Print and shaded views of the part. All mm, measured from the part's lowest x, y and z. Coordinates: 2 decimals unless noted, no trailing zeros. Order: outer loops, then holes, each group sorted by start corner. A loop starts at its lowest first (then second) coordinate and runs counter-clockwise, first axis right, second up. Notation, with made-up numbers: (0.5, 42.25) -> (26.5, 42.25) arc R27 cw to (26.5, 81.25) -> close; hole circle Ø4 at (-23.75, 34.25). An arc over 180 degrees is marked (long way). Return JSON: item names as keys, results as strings. Group by question number.
1) Cut at D-D (z = 4). Write the cut outline in (x, y).
2) Cut at C-C (y = 0.2). State how many separate pieces and enclosed holes the cut face has, and give its area (3 significant figures).
3) Probe line 1 (Z direction, x = 10.5, y = 0.65); line 2 (Z direction, x = 36, y = 0.9). List the from-to ranges inside material, lowest first.
4) Cut at A-A (z = 12.5). Write the cut outline in (x, y).
5) Cut at B-B (x = 6). Write the cut outline in (y, z).
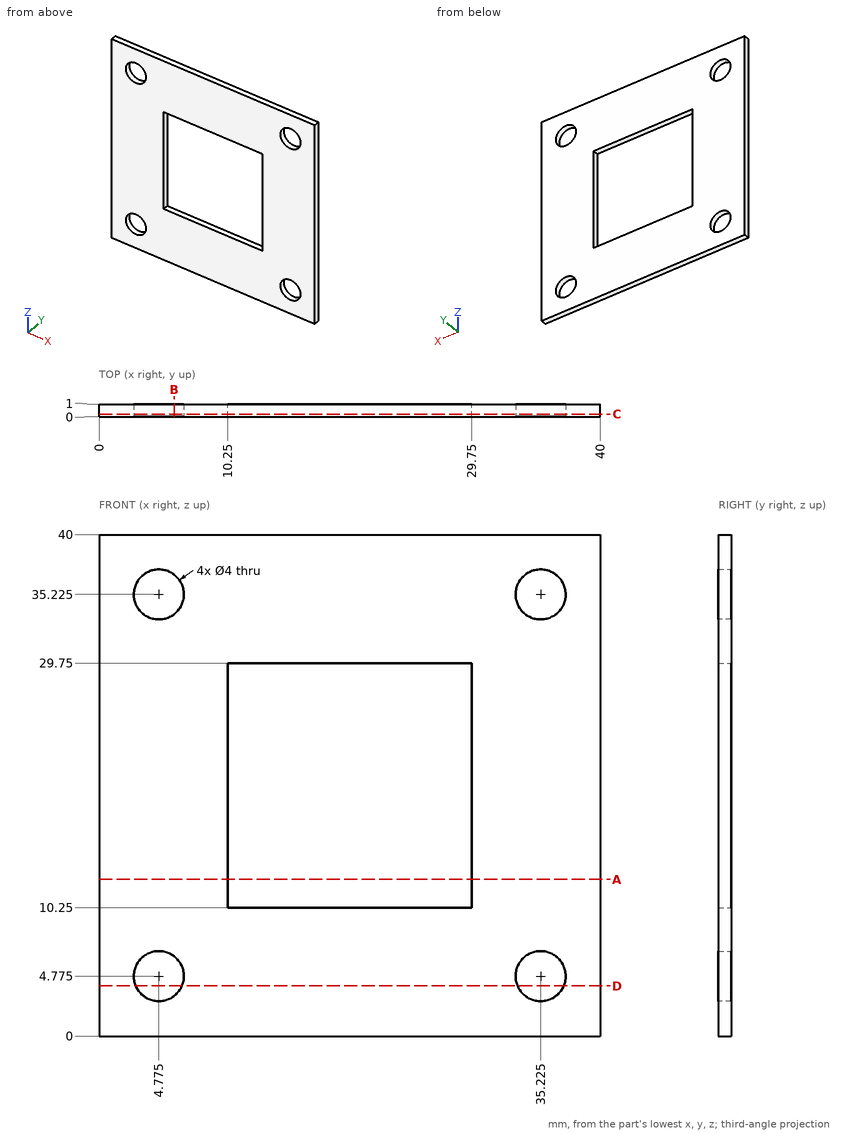
Answers below:
{
 "1": {"outline": "(0, 0) -> (2.93, 0) -> (2.93, 1) -> (0, 1) -> close; (6.62, 0) -> (33.38, 0) -> (33.38, 1) -> (6.62, 1) -> close; (37.07, 0) -> (40, 0) -> (40, 1) -> (37.07, 1) -> close"},
 "2": {"separate pieces": "1", "enclosed holes": "5", "area": "1,170 mm^2"},
 "3": {"line 1": "z = 0 to 10.25, 29.75 to 40", "line 2": "z = 0 to 2.93, 6.62 to 33.38, 37.07 to 40"},
 "4": {"outline": "(0, 0) -> (10.25, 0) -> (10.25, 1) -> (0, 1) -> close; (29.75, 0) -> (40, 0) -> (40, 1) -> (29.75, 1) -> close"},
 "5": {"outline": "(0, 0) -> (1, 0) -> (1, 3.19) -> (0, 3.19) -> close; (0, 6.36) -> (1, 6.36) -> (1, 33.64) -> (0, 33.64) -> close; (0, 36.81) -> (1, 36.81) -> (1, 40) -> (0, 40) -> close"}
}
